from build123d import *

# Parameters (mm, degrees)
SKETCH1_W                                       = 16
SKETCH1_H                                       = 16
SKETCH1_W_2                                     = 14
SKETCH1_H_2                                     = 14
BOSS_EXTRUDE1_DEPTH                             = 50
SKETCH2_R                                       = 4.25
CUT_EXTRUDE1_DEPTH                              = 54.103672189
CSK_FOR_M3_FLAT_HEAD_MACHINE_SCREW1_D           = 3.4
CSK_FOR_M3_FLAT_HEAD_MACHINE_SCREW1_CSINK_D     = 6.3
CSK_FOR_M3_FLAT_HEAD_MACHINE_SCREW1_CSINK_ANGLE = 90


with BuildPart() as part:
    # Sketch1 → Boss-Extrude1 (new body)
    with BuildSketch(Plane.XY):
        Rectangle(SKETCH1_W, SKETCH1_H)
        Rectangle(SKETCH1_W_2, SKETCH1_H_2, mode=Mode.SUBTRACT)
    extrude(amount=BOSS_EXTRUDE1_DEPTH)

    # Sketch2 → Cut-Extrude1 (cut, through all)
    with BuildSketch(Plane(origin=(0, 8, 0), x_dir=(1, 0, 0), z_dir=(0, 1, 0))):
        with Locations(Location((0, -9.5, 0), (0, 0, 270))):
            Circle(SKETCH2_R)
    extrude(amount=-CUT_EXTRUDE1_DEPTH, mode=Mode.SUBTRACT)

    # CSK for M3 Flat Head Machine Screw1 (through all)
    with Locations(Plane(origin=(0, 8, 20.5), x_dir=(0, 0, 1), z_dir=(0, 1, 0))):
        with Locations((0, 0)):
            csk_for_m3_flat_head_machine_screw1 = CounterSinkHole(CSK_FOR_M3_FLAT_HEAD_MACHINE_SCREW1_D / 2, CSK_FOR_M3_FLAT_HEAD_MACHINE_SCREW1_CSINK_D / 2, counter_sink_angle=CSK_FOR_M3_FLAT_HEAD_MACHINE_SCREW1_CSINK_ANGLE)

    # Mirror1: CSK for M3 Flat Head Machine Screw1 across plane
    add(csk_for_m3_flat_head_machine_screw1.mirror(Plane.ZX), mode=Mode.SUBTRACT)


solid = part.part
Can you work these out from the model? Positions are in its coordinate system, mm. A direction names the side the tool comes from. Give positions to 0.01 mm unless a question says otherwise; leave off trailing zeros. Loops run counter-clockwise (first coordinate to the right, second up) from the corner with the lowest first, then second, coordinate; pieces in that order, holes last. Notation, with made-up numbers: (20.5, -18.75) - (25.5, -18.75) arc R16 ccw to (25.5, -12.75) - close; hole circle Ø7 at (40, 61). An arc over 180 degrees is marked (long way). Answer as a JSON object with one key per item and string values.
Q1. Which directions (+Z, -Z, +X, -X, +Y, -Y) give clear straight access to the entire face, cutting with the end or side of a thin tool? Please do faces 4 (the flat face through (0, -7, 25)), 5 (the flat face through (8, 0, 25)).
Geometry says:
{"face 4": "+Z, -Z", "face 5": "+Z, -Z, +X, +Y, -Y"}
Q2. Imagine slicing it at A-A on x = 3.75. Write out the boundary of the cut face in (y, z).
Geometry says:
{"outline": "(-8, 0) - (-7, 0) - (-7, 7.5) - (-8, 7.5) - close; (-8, 11.5) - (-7, 11.5) - (-7, 50) - (-8, 50) - close; (7, 0) - (8, 0) - (8, 7.5) - (7, 7.5) - close; (7, 11.5) - (8, 11.5) - (8, 50) - (7, 50) - close"}
Q3. If I drill on L1, parallel to X at y = -7.45, z = 9.5; L2, parallel to X at y = -1.25, z = 13, over which ranges is the centre line in solid material (lowest first)?
Geometry says:
{"L1": "-8 to -4.25, 4.25 to 8", "L2": "-8 to -7, 7 to 8"}
Q4. Imagine slicing it at D-D on x = 0. Write out the boundary of the cut face in (y, z).
Geometry says:
{"outline": "(-8, 0) - (-7, 0) - (-7, 5.25) - (-8, 5.25) - close; (-8, 13.75) - (-7, 13.75) - (-7, 18.35) - (-8, 17.35) - close; (-8, 23.65) - (-7, 22.65) - (-7, 50) - (-8, 50) - close; (7, 0) - (8, 0) - (8, 5.25) - (7, 5.25) - close; (7, 13.75) - (8, 13.75) - (8, 17.35) - (7, 18.35) - close; (7, 22.65) - (8, 23.65) - (8, 50) - (7, 50) - close"}
Q5. Imagine slicing it at C-C on y = 4. Write out the boundary of the cut face in (x, z), plus the area to 3 significant figures.
Geometry says:
{"outline": "(-8, 0) - (-7, 0) - (-7, 50) - (-8, 50) - close; (7, 0) - (8, 0) - (8, 50) - (7, 50) - close", "area": "100 mm²"}
Q6. Imagine slicing it at B-B on z = 20.5. Write out the boundary of the cut face in (x, y).
Geometry says:
{"outline": "(-8, -8) - (-3.15, -8) - (-2.15, -7) - (-7, -7) - (-7, 7) - (-2.15, 7) - (-3.15, 8) - (-8, 8) - close; (2.15, -7) - (3.15, -8) - (8, -8) - (8, 8) - (3.15, 8) - (2.15, 7) - (7, 7) - (7, -7) - close"}
Q7. Will this pin go through, and if not, where does the flat tip stop? P1, Ø5, axis at x = 4, y = -5.5, coming from the -Z side.
Geometry says:
{"P1": "z = 0"}
Q8. If we mould it in two halves opening along Z, with no side actions, what happens to faces 1 (the cylindrical face through (0.187, 7.507, 5.254)), 2 (the flat face through (-7.15, 0.04, 0)), 3 (the flat face through (-7, 0, 25))? For each: pulls with the +Z half, pulls with the -Z half, needs draft (parallel to the pull), parting line crosses it, or undercut.
Geometry says:
{"face 1": "undercut", "face 2": "pulls with the -Z half", "face 3": "needs draft"}
